```python
from build123d import *

# Parameters (mm, degrees)
F0_W            = 42.8
F0_H            = 42.8
F1_DEPTH        = 650
F3_D            = 5
F3_DEPTH        = 15
F3_TIP          = 1.5021515476
F3_COPIES_COUNT = 4


# Not quite as in the source:
# - a pattern or mirror of a feature is missing from the dataset's text; its kind, count and spacing are read off the source's solid


with BuildPart() as f1:
    # F0 (on Top) → F1 (new body)
    with BuildSketch(Plane.XY):
        with BuildLine():
            Line((-0.3117055804, 27.0466537178), (-46.1117055804, 27.0466537178))
            ThreePointArc((-46.1117055804, 27.0466537178), (-47.8794725333, 26.3144206707), (-48.6117055804, 24.5466537178))
            Line((-48.6117055804, 24.5466537178), (-48.6117055804, -21.2533462822))
            ThreePointArc((-48.6117055804, -21.2533462822), (-47.8794725333, -23.0211132352), (-46.1117055804, -23.7533462822))
            Line((-46.1117055804, -23.7533462822), (-0.3117055804, -23.7533462822))
            ThreePointArc((-0.3117055804, -23.7533462822), (1.4560613726, -23.0211132352), (2.1882944196, -21.2533462822))
            Line((2.1882944196, -21.2533462822), (2.1882944196, 24.5466537178))
            ThreePointArc((2.1882944196, 24.5466537178), (1.4560613726, 26.3144206707), (-0.3117055804, 27.0466537178))
        make_face()
        with Locations((-23.2117055804, 1.6466537178)):
            Rectangle(F0_W, F0_H, mode=Mode.SUBTRACT)
    extrude(amount=F1_DEPTH)

    # F3
    with Locations(Plane.XZ.offset(23.7533462822)):
        with Locations((-23.2117055804, 644.05)):
            f3 = Hole(F3_D / 2, depth=F3_DEPTH)
            with Locations((0, 0, -(F3_DEPTH + F3_TIP / 2))):  # 118° drill point
                Cone(0, F3_D / 2, F3_TIP, mode=Mode.SUBTRACT)

    # F3_copies: F3 ×4 about axis
    f3_copies_axis = Axis((-23.211706, 1.646654, 0), (0, 0, 1))
    for i in range(1, F3_COPIES_COUNT):
        add(f3.rotate(f3_copies_axis, i * 360 / F3_COPIES_COUNT), mode=Mode.SUBTRACT)


solid = f1.part
```
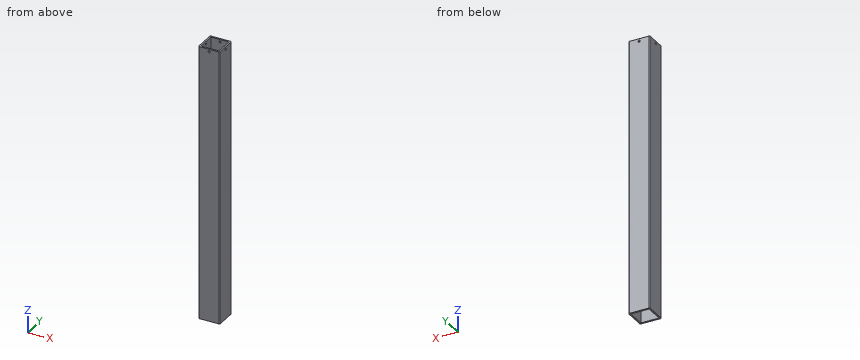
Design review of the part built by this model. Coordinates are the model's own, in mm. Coordinates: 2 decimals unless noted, no trailing zeros. Write each loop counter-clockwise with the first axis right and the second up, starting at its lowest first coordinate (ties: lowest second). Pieces come first, ordered by that corner, then holes.
1) Add section A-A (x = -34.5). Write out the cut boundary in (y, z), plus the area to 3 significant figures.
2) To check wall thickness, follow L1, parallel to X at y = -10, z = 254; L2, parallel to X at y = 25, z = 644; L3, parallel to Y at x = -40.5, z = 388. State the ranges of each line that lie inside material, in increasing order.
3) Insertion check: pin 1 (6 mm diameter, centred on x = -23.21, z = 644.05, fed in from -Y). The pin has a flat end and moves straight along its axis. Give the tip position at first contact, or say it passes through.
4) Add section C-C (y = 9.5). Write out the cut boundary in (x, z).
5) Add section B-B (z = 63). Write out the cut boundary in (x, y), plus the area to 3 significant figures.
Check result:
1. outline: (-23.75, 0) - (-19.75, 0) - (-19.75, 650) - (-23.75, 650) - close; (23.05, 0) - (27.05, 0) - (27.05, 650) - (23.05, 650) - close
1. area: 5,200 mm2
2. L1: x = -48.61 to -44.61, -1.81 to 2.19
2. L2: x = -48.57 to -25.71, -20.71 to 2.15
2. L3: y = -23.75 to -19.75, 23.05 to 27.05
3. pin 1: stops at y = -23.75
4. outline: (-48.61, 0) - (-44.61, 0) - (-44.61, 650) - (-48.61, 650) - close; (-1.81, 0) - (2.19, 0) - (2.19, 650) - (-1.81, 650) - close
5. outline: (-48.61, -21.25) arc R2.5 ccw to (-46.11, -23.75) - (-0.31, -23.75) arc R2.5 ccw to (2.19, -21.25) - (2.19, 24.55) arc R2.5 ccw to (-0.31, 27.05) - (-46.11, 27.05) arc R2.5 ccw to (-48.61, 24.55) - close; hole (-44.61, -19.75) - (-1.81, -19.75) - (-1.81, 23.05) - (-44.61, 23.05) - close
5. area: 743 mm2
